The listing builds one solid part. Answer for the finished solid, in the listing's coordinates (mm). Face numbers are marked on the shaded views. A direction names the side the tool comes from. Coordinates: 2 decimals unless noted, no trailing zeros. Order: outer loops, then holes, each group sorted by start corner. A loop starts at its lowest first (then second) coordinate and runs counter-clockwise, first axis right, second up. Notation, with made-up numbers: (-25.5, 61) - (7.5, 61) arc R24 ccw to (7.5, 95) - close; hole circle Ø6 at (43.25, 20). An arc over 180 degrees is marked (long way). Use one line per item in the form item = value. Start each with the question number.
Item 1: A tool of negligible diameter and unlimited length cuts with its end or side. For the marked faces 1 and 2, from which of +Z, -Z, +X, -X, +Y, -Y can it reach the whole face along a straight path? Write none if from no direction.
Item 2: Consider line 1 along Y through (x, z) = (-18.5, 13); line 2 along X through (y, z) = (-31, 3). Determine where each line is inside the solid, lowest interval first. Write a range as [from, to].
Item 3: Section B-B, the plane x = 2 is taken. Write down the section's boundary in (y, z), and give its area (3 significant figures).
Item 4: Section A-A, the plane z = 5 is taken. Write down the section's boundary in (x, y).
Item 5: Section C-C, the plane y = -25 is taken. Write down the section's boundary in (x, z), and give its area (3 significant figures).
Item 6: Each of these flat-tipped pins is pushed along its axis until it touches: pin 1 Ø1 at (x, z) = (-4, -6.5) entering from -Y; pin 2 Ø12 at (y, z) = (-9.5, -4.5) entering from +X. Where does it stop, or does it pass through?
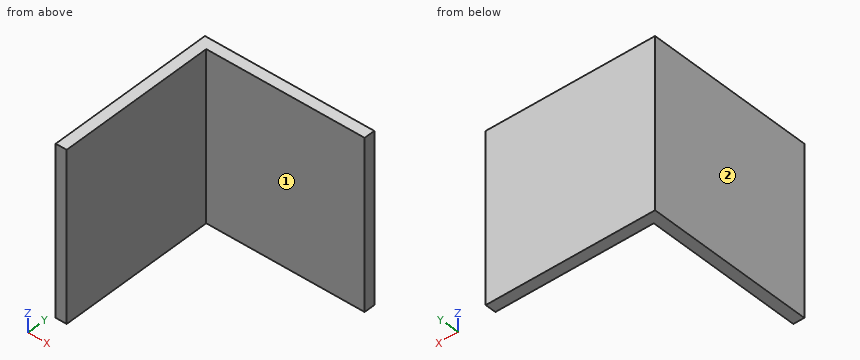
from build123d import *

# Parameters (mm, degrees)
F0_W     = 33.02
F0_H     = 33.02
F1_DEPTH = 33.02
F2_T     = -2.1336


with BuildPart() as f1:
    # F0 (on Front) → F1 (new body)
    with BuildSketch(Plane.XZ):
        with Locations((-4.376881, 3.478918)):
            Rectangle(F0_W, F0_H)
    extrude(amount=F1_DEPTH)

    # F2
    f2_openings = [f1.faces().sort_by_distance(p)[0] for p in [
        (-4.376881, -16.51, -13.031082),
        (12.133119, -16.51, 3.478918),
        (-4.376881, -33.02, 3.478918),
        (-4.376881, -16.51, 19.988918),
    ]]
    offset(amount=F2_T, openings=f2_openings)


solid = f1.part
Response:
q1.face_1 = +Z, -Z, +X, -Y
q1.face_2 = +Z, -Z, -X, +Y, -Y
q2.line_1 = [-2.13, 0]
q2.line_2 = [-20.89, -18.75]
q3.outline = (-2.13, -13.03) - (0, -13.03) - (0, 19.99) - (-2.13, 19.99) - close
q3.area = 70.5 mm2
q4.outline = (-20.89, -33.02) - (-18.75, -33.02) - (-18.75, -2.13) - (12.13, -2.13) - (12.13, 0) - (-20.89, 0) - close
q5.outline = (-20.89, -13.03) - (-18.75, -13.03) - (-18.75, 19.99) - (-20.89, 19.99) - close
q5.area = 70.5 mm2
q6.pin_1 = -2.13
q6.pin_2 = -18.75
